from build123d import *

# Parameters (mm, degrees)
SKETCH_R      = 0.75
PAD_DEPTH     = 5
SKETCH001_W   = 6.7
SKETCH001_H   = 19.2
SKETCH001_W_2 = 2.7
SKETCH001_H_2 = 15.2
SKETCH001_W_3 = 19.2
SKETCH001_H_3 = 6.7
SKETCH001_W_4 = 15.2
SKETCH001_H_4 = 2.7
PAD001_DEPTH  = 5
CHAMFER_SIZE  = 1


with BuildPart() as part:
    # Sketch → Pad (new body)
    with BuildSketch(Plane.XY):
        with BuildLine():
            Line((0, 0), (40, 0))
            Line((40, 0), (40, 37))
            ThreePointArc((40, 37), (39.12132, 39.12132), (37, 40))
            Line((37, 40), (0, 40))
            Line((0, 40), (0, 0))
        make_face()
        with Locations((5, 5)):
            Circle(SKETCH_R, mode=Mode.SUBTRACT)
        with Locations((25.33016, 25.33016)):
            Circle(SKETCH_R, mode=Mode.SUBTRACT)
    extrude(amount=PAD_DEPTH)

    # Sketch001 (on Face9 of Pad) → Pad001 (join)
    with BuildSketch(Plane.XY.offset(5)):
        with Locations((3.78016, 25.33016)):
            Rectangle(SKETCH001_W, SKETCH001_H)
        with Locations((3.78016, 25.33016)):
            Rectangle(SKETCH001_W_2, SKETCH001_H_2, mode=Mode.SUBTRACT)
        with Locations((25.33016, 3.78016)):
            Rectangle(SKETCH001_W_3, SKETCH001_H_3)
        with Locations((25.33016, 3.78016)):
            Rectangle(SKETCH001_W_4, SKETCH001_H_4, mode=Mode.SUBTRACT)
    extrude(amount=PAD001_DEPTH)

    # Chamfer
    chamfer_edges = [part.edges().sort_by_distance(p)[0] for p in [
        (25.33016, 2.43016, 10),
        (17.73016, 3.78016, 10),
        (25.33016, 5.13016, 10),
        (32.93016, 3.78016, 10),
        (5.13016, 25.33016, 10),
        (3.78016, 17.73016, 10),
        (2.43016, 25.33016, 10),
        (3.78016, 32.93016, 10),
    ]]
    chamfer(chamfer_edges, length=CHAMFER_SIZE)


solid = part.part
Geometry: final body of the model. Coordinates: model frame, mm. A direction names the side the tool comes from. Round coordinates to 2 decimals unless told otherwise and drop trailing zeros. Loops run counter-clockwise (first coordinate to the right, second up) from the corner with the lowest first, then second, coordinate; pieces in that order, holes last.
Q1. Section A-A on z = 5.5. Return loops of the section in (x, y), plus the area to 3 significant figures.
Q2. Pin query (flat end, axial travel): P1, Ø1.4, axis at y = 4.5, z = 7.5, coming from the -X side; P2, Ø2.5, axis at x = 3.5, z = 8.5, coming from the +Y side; P3, Ø0.8, axis at x = 27, y = 4.5, coming from the +Z side. Return the tip coordinate at first contact, or that it passes through.
Q3. Section C-C on z = 9.5. Return loops of the section in (x, y).
Q4. Access query for faces 1 (the flat face through (0.43, 25, 7)), 2 (the flat face through (25, 0.43, 7)), 3 (the flat face through (25, 4, 5)), 4 (the flat face through (7.13, 25, 7)). Directions: +Z, -Z, +X, -X, +Y, -Y. A direction counts if a zero-diameter tool reaches every point of the face in a straight line with its end or side. Return the directions, or none.
Q5. Section D-D on y = 11. Return loops of the section in (x, z).
Q6. Pull-direction query (Y, two-part tool) for faces 5 (the flat face through (25, 7.13, 7)), 6 (the flat face through (34.93, 4, 7)), 7 (the flat face through (1.94, 25.21, 9.49)); classes: released by +Y, released by -Y, zero draft, split by the parting line, or undercut.
Q7. Section B-B on y = 19.5. Return loops of the section in (x, z), plus the area to 3 significant figures.
Q8. Material intervals for L1, parallel to Y at x = 5, z = 3.45; L2, parallel to X at y = 20.5, z = 8.5, sorted ascending.
Evaluation:
1. outline: (0.43, 15.73) - (7.13, 15.73) - (7.13, 34.93) - (0.43, 34.93) - close; (15.73, 0.43) - (34.93, 0.43) - (34.93, 7.13) - (15.73, 7.13) - close; hole (2.43, 17.73) - (5.13, 17.73) - (5.13, 32.93) - (2.43, 32.93) - close; hole (17.73, 2.43) - (32.93, 2.43) - (32.93, 5.13) - (17.73, 5.13) - close
1. area: 175 mm2
2. P1: stops at x = 15.73
2. P2: stops at y = 34.93
2. P3: stops at z = 5
3. outline: (0.43, 15.73) - (7.13, 15.73) - (7.13, 34.93) - (0.43, 34.93) - close; (15.73, 0.43) - (34.93, 0.43) - (34.93, 7.13) - (15.73, 7.13) - close; hole (1.93, 17.23) - (5.63, 17.23) - (5.63, 33.43) - (1.93, 33.43) - close; hole (17.23, 1.93) - (33.43, 1.93) - (33.43, 5.63) - (17.23, 5.63) - close
4. face 1: +Z, -X, +Y, -Y
4. face 2: +Z, +X, -X, -Y
4. face 3: +Z
4. face 4: +Z, +X, +Y, -Y
5. outline: (0, 0) - (40, 0) - (40, 5) - (0, 5) - close
6. face 5: released by +Y
6. face 6: zero draft
6. face 7: undercut
7. outline: (0, 0) - (40, 0) - (40, 5) - (7.13, 5) - (7.13, 10) - (6.13, 10) - (5.13, 9) - (5.13, 5) - (2.43, 5) - (2.43, 9) - (1.43, 10) - (0.43, 10) - (0.43, 5) - (0, 5) - close
7. area: 219 mm2
8. L1: y = 0 to 4.25, 5.75 to 40
8. L2: x = 0.43 to 2.43, 5.13 to 7.13
